Build history of the part. All positions in model axes, mm. Round coordinates to 2 decimals unless told otherwise and drop trailing zeros. Loops run counter-clockwise (first coordinate to the right, second up) from the corner with the lowest first, then second, coordinate; pieces in that order, holes last. Notation, with made-up numbers: M 12,10 L 55,10 A26 cw 55,37 Z; hole C -3.75,38 d11. An arc over 180 degrees is marked long. One line per item, written item: value.
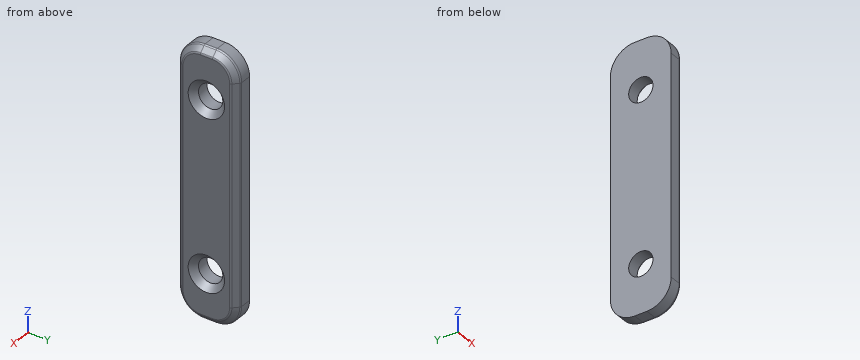
```python
from build123d import *

# Parameters (mm, degrees)
BOSS_EXTRUDE1_DEPTH = 3
CHAMFER1_SIZE       = 1
FILLET1_R           = 0.4
SKETCH2_R           = 2
CUT_EXTRUDE1_DEPTH  = 3
CHAMFER2_SIZE       = 1


with BuildPart() as part:
    # Sketch1 → Boss-Extrude1 (new body)
    with BuildSketch(Plane(origin=(0, 0, 0), x_dir=(0, 0, -1), z_dir=(1, 0, 0))):
        with BuildLine():
            Line((-18, -5), (18, -5))
            ThreePointArc((18, -5), (20.828427125, -3.828427125), (22, -1))
            Line((22, -1), (22, 1))
            ThreePointArc((22, 1), (20.828427125, 3.828427125), (18, 5))
            Line((18, 5), (-18, 5))
            ThreePointArc((-18, 5), (-20.828427125, 3.828427125), (-22, 1))
            Line((-22, 1), (-22, -1))
            ThreePointArc((-22, -1), (-20.828427125, -3.828427125), (-18, -5))
        make_face()
    extrude(amount=BOSS_EXTRUDE1_DEPTH)

    # Chamfer1
    chamfer1_edges = [part.edges().sort_by_distance(p)[0] for p in [
        (3, 3.828427125, 20.828427125),
        (3, 0, 22),
        (3, -3.828427125, 20.828427125),
        (3, -5, 0),
        (3, -3.828427125, -20.828427125),
        (3, 0, -22),
        (3, 3.828427125, -20.828427125),
        (3, 5, 0),
    ]]
    chamfer(chamfer1_edges, length=CHAMFER1_SIZE)

    # Fillet1
    fillet1_edges = [part.edges().sort_by_distance(p)[0] for p in [
        (3, 3.121320344, -20.121320344),
        (3, 4, 0),
        (3, 3.121320344, 20.121320344),
        (3, 0, 21),
        (3, -3.121320344, 20.121320344),
        (3, -4, 0),
        (3, -3.121320344, -20.121320344),
        (3, 0, -21),
        (2, 0, -22),
        (2, -3.828427125, -20.828427125),
        (2, -5, 0),
        (2, -3.828427125, 20.828427125),
        (2, 0, 22),
        (2, 3.828427125, 20.828427125),
        (2, 5, 0),
        (2, 3.828427125, -20.828427125),
    ]]
    fillet(fillet1_edges, radius=FILLET1_R)

    # Sketch2 → Cut-Extrude1 (cut)
    with BuildSketch(Plane(origin=(3, 0, 0), x_dir=(0, 0, -1), z_dir=(1, 0, 0))):
        with Locations((-14, 0)):
            Circle(SKETCH2_R)
        with Locations((14, 0)):
            Circle(SKETCH2_R)
    extrude(amount=-CUT_EXTRUDE1_DEPTH, mode=Mode.SUBTRACT)

    # Chamfer2
    chamfer2_edges = [part.edges().sort_by_distance(p)[0] for p in [
        (3, 0, 16),
        (3, 0, -12),
    ]]
    chamfer(chamfer2_edges, length=CHAMFER2_SIZE)


solid = part.part
```
Item 1: Slice it at B-B, the plane z = 14. Give the cut face in (x, y), and give its area (3 significant figures).
Check values:
outline: M 0,-5 L 1.83,-5 A0.4 ccw 2.12,-4.88 L 2.88,-4.12 A0.4 ccw 3,-3.83 L 3,-3 L 2,-2 L 0,-2 Z; M 0,2 L 2,2 L 3,3 L 3,3.83 A0.4 ccw 2.88,4.12 L 2.12,4.88 A0.4 ccw 1.83,5 L 0,5 Z
area: 16.0 mm2
Item 2: Slice it at A-A, the plane x = 0.65. Give the cut face in (y, z), and give its area (3 significant figures).
Check values:
outline: M -5,-18 A4 ccw -1,-22 L 1,-22 A4 ccw 5,-18 L 5,18 A4 ccw 1,22 L -1,22 A4 ccw -5,18 Z; hole C 0,-14 d4; hole C 0,14 d4
area: 401 mm2
Item 3: Wall check: line 1 along Y through (x, z) = (0.65, -14); line 2 along Z through (x, y) = (1.2, 1.5); line 3 along Y through (x, z) = (2.7, -12.5) (3 decimals). Give the ranges that are in metal, low to high.
Check values:
line 1: y = -5 to -2, 2 to 5
line 2: z = -21.97 to -15.32, -12.68 to 12.68, 15.32 to 21.97
line 3: y = -4.3 to -2.245, 2.245 to 4.3
Item 4: Slice it at C-C, the plane y = 0. Give the cut face in (x, z), and give its area (3 significant figures).
Check values:
outline: M 0,-22 L 1.83,-22 A0.4 ccw 2.12,-21.88 L 2.88,-21.12 A0.4 ccw 3,-20.83 L 3,-17 L 2,-16 L 0,-16 Z; M 0,-12 L 2,-12 L 3,-11 L 3,11 L 2,12 L 0,12 Z; M 0,16 L 2,16 L 3,17 L 3,20.83 A0.4 ccw 2.88,21.12 L 2.12,21.88 A0.4 ccw 1.83,22 L 0,22 Z
area: 105 mm2
Item 5: Slice it at D-D, the plane z = -2. Give the cut face in (x, y), and give its area (3 significant figures).
Check values:
outline: M 0,-5 L 1.83,-5 A0.4 ccw 2.12,-4.88 L 2.88,-4.12 A0.4 ccw 3,-3.83 L 3,3.83 A0.4 ccw 2.88,4.12 L 2.12,4.88 A0.4 ccw 1.83,5 L 0,5 Z
area: 29.0 mm2
